Design review of the part built by this model. Coordinates are the model's own, in mm. Face numbers are marked on the shaded views. Coordinates: 2 decimals unless noted, no trailing zeros. Write each loop counter-clockwise with the first axis right and the second up, starting at its lowest first coordinate (ties: lowest second). Pieces come first, ordered by that corner, then holes. Notation, with made-up numbers: M -4,-0.5 L 3,-0.5 A25 cw 3,11.5 Z; hole C 34.25,81.25 d8. An arc over 180 degrees is marked long. One line per question, with ' | ' between items.
from build123d import *

# Parameters (mm, degrees)
F0_W      = 150
F0_H      = 150
F1_DEPTH  = 40
F2_W      = 145
F2_H      = 145
F3_DEPTH  = 135
F6_D      = 20
F6_DEPTH  = 5
F6_TIP    = 6.0086061903
F7_W      = 150
F7_H      = 150
F8_DEPTH  = 5
F10_D     = 12
F10_DEPTH = 5
F10_TIP   = 3.6051637142


with BuildPart() as f1:
    # F0 (on Top) → F1 (new body)
    with BuildSketch(Plane.XY):
        with Locations((39.0263837129, 41.0243682017)):
            Rectangle(F0_W, F0_H)
    extrude(amount=F1_DEPTH)

    # F2 (on face) → F3 (cut)
    with BuildSketch(Plane.XY.offset(40)):
        with Locations((39.0263837129, 41.0243682017)):
            Rectangle(F2_W, F2_H)
    extrude(amount=-F3_DEPTH, mode=Mode.SUBTRACT)

    # F6
    with Locations(Plane(origin=(0, 116.0243682017, 0), x_dir=(-1, 0, 0), z_dir=(0, 1, 0))):
        with Locations((-39.0263837129, 15.2529580519), (-10.3633506224, 15.2529580519)):
            Hole(F6_D / 2, depth=F6_DEPTH)
            with Locations((0, 0, -(F6_DEPTH + F6_TIP / 2))):  # 118° drill point
                Cone(0, F6_D / 2, F6_TIP, mode=Mode.SUBTRACT)

    # F7 (on Top) → F8 (join)
    with BuildSketch(Plane.XY):
        with Locations((38.9731861651, 41.1050692201)):
            Rectangle(F7_W, F7_H)
    extrude(amount=F8_DEPTH)

    # F10
    with Locations(Plane.YZ.offset(114.0263837129)):
        with Locations((59.0243682017, 32.5), (41.0243682017, 25)):
            Hole(F10_D / 2, depth=F10_DEPTH)
            with Locations((0, 0, -(F10_DEPTH + F10_TIP / 2))):  # 118° drill point
                Cone(0, F10_D / 2, F10_TIP, mode=Mode.SUBTRACT)


solid = f1.part
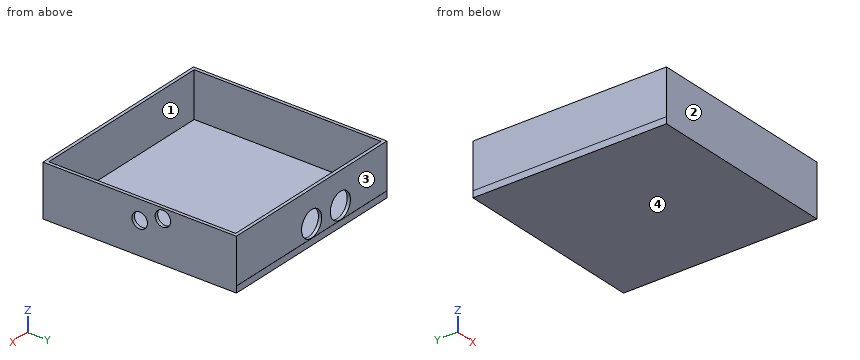
1. To check wall thickness, follow line 1 along Y through (x, z) = (65, 26.5); line 2 along X through (y, z) = (14, 37.5); line 3 along Z through (x, y) = (27, 75). State the ranges of each line that lie inside material, in increasing order. Write a range as [from, to].
Answer sheet:
line 1: [-33.98, -31.48], [113.52, 116.02] | line 2: [-35.97, -33.47], [111.53, 114.03] | line 3: [0, 5]
2. Take a section at B-B (x = 34). Write out the cut boundary in (y, z), then the cut area to 3 significant figures.
Answer sheet:
outline: M -33.98,0 L 116.11,0 L 116.11,5 L 116.02,5 L 116.02,6.61 L 113.52,6.61 L 113.52,5 L -31.48,5 L -31.48,40 L -33.98,40 Z; M 113.52,23.9 L 116.02,23.9 L 116.02,40 L 113.52,40 Z | area: 882 mm^2
3. Take a section at C-C (z = 11.5). Write out the cut boundary in (x, y), then the cut area to 3 significant figures.
Answer sheet:
outline: M -35.97,-33.98 L 114.03,-33.98 L 114.03,116.02 L 48.3,116.02 L 48.3,113.52 L 111.53,113.52 L 111.53,-31.48 L -33.47,-31.48 L -33.47,113.52 L 1.09,113.52 L 1.09,116.02 L -35.97,116.02 Z; M 19.63,113.52 L 29.76,113.52 L 29.76,116.02 L 19.63,116.02 Z | area: 1,380 mm^2
4. Draft analysis for pull direction Y (two halves, no side actions). For the marked faces 1, 2, 3 and 4, state which applies: pulls with the +Y half, pulls with the -Y half, needs draft (parallel to the pull), parting line crosses it, or undercut.
Answer sheet:
face 1: undercut | face 2: pulls with the -Y half | face 3: pulls with the +Y half | face 4: needs draft
5. Take a section at A-A (y = 2). Write out the cut boundary in (x, z), then the cut area to 3 significant figures.
Answer sheet:
outline: M -36.03,0 L 114.03,0 L 114.03,40 L 111.53,40 L 111.53,5 L -33.47,5 L -33.47,40 L -35.97,40 L -35.97,5 L -36.03,5 Z | area: 925 mm^2
6. Take a section at D-D (x = -9). Write out the cut boundary in (y, z).
Answer sheet:
outline: M -33.98,0 L 116.11,0 L 116.11,5 L 116.02,5 L 116.02,40 L 113.52,40 L 113.52,5 L -31.48,5 L -31.48,40 L -33.98,40 Z
7. Insertion check: pin 1 Ø4 at (x, y) = (41, 9.5) entering from +Z; pin 2 Ø14 at (y, z) = (59.02, 32.5) entering from -X; pin 3 Ø10.5 at (x, z) = (17.5, 16) entering from +Y. Each pin has a flat end and moves straight along its axis. Give the tip position at first contact, or say it passes through.
Answer sheet:
pin 1: z = 5 | pin 2: x = -35.97 | pin 3: y = 116.02
